Could you check a few things on this model? Use its own coordinates, in mm. A direction names the side the tool comes from. Coordinates: 2 decimals unless noted, no trailing zeros. Order: outer loops, then holes, each group sorted by start corner. A loop starts at its lowest first (then second) coordinate and runs counter-clockwise, first axis right, second up. Notation, with made-up numbers: (21, -33) -> (40, -33) arc R25 cw to (40, -21) -> close; hole circle Ø5 at (86.5, 51). An arc over 180 degrees is marked (long way). Put each result on its own line as item: value. Start each with the question number.
Q1. Please list where these lines run through material, in increasing order: line 1 along X through (y, z) = (-3, 7); line 2 along Z through (x, y) = (-6.5, -35.5); line 3 along X through (y, z) = (-43, 9).
Q2. For faces 4 (the face through (-23.2, 23.5, 10)), 5 (the face through (-40.1, 5, 2.7)), 6 (the face through (-46.6, 0.07, 9.14)), which set-ups out of +Z, -Z, +X, -X, +Y, -Y let a thin tool reach every point of the face, with its end or its side?
Q3. If we section it at B-B (x = 0): Please give me the cut outline in (y, z), and give its area (3 significant figures).
Q4. If we section it at D-D (x = 42): Please give me the cut outline in (y, z).
Q5. Will these pins go through, and if not, where does the flat tip stop? pin 1 (4 mm diameter, centred on x = -15, z = 8, fed in from +Y); pin 2 (8 mm diameter, centred on y = -42.33, z = 5, fed in from -X); pin 3 (8 mm diameter, centred on x = 21.5, z = 15, fed in from +Y); pin 4 (5.5 mm diameter, centred on x = 42.33, z = 5, fed in from -Y).
Q6. If we section it at A-A (z = 5): Count the separate pieces of the cut face and the enclosed holes in it, and give its area (3 significant figures).
Q7. We'd pull the mould along X, two halves only. Please class faces 1 (the face through (-0.07, 39.47, 5.9)), 2 (the face through (-25.14, -24.22, 12.07)), 3 (the face through (-20.98, -28.05, 13.45)): +X half, -X half, draft (parallel to the pull), parting line (faces both ways), or undercut.
from build123d import *
from build123d.topology import SkipClean

# Parameters (mm, degrees)
CROQUIS1_R                 = 32.5
SALIENTE_EXTRUIR1_DEPTH    = 10
CROQUIS2_R                 = 3
CORTAR_EXTRUIR1_DEPTH      = 72.50174823
MATRIZC1_COUNT             = 4
SALIENTE_EXTRUIR2_DEPTH    = 10
CORTAR_EXTRUIR2_DEPTH      = 71.089228844
CORTAR_EXTRUIR2_DEPTH_BACK = 71.089228844
CROQUIS4_R                 = 3
REDONDEO1_R                = 3
SIMETR_A3_START            = 32.113081288
SIMETR_A3_DEPTH            = 5.333547499
SIMETR_A3_START_2          = -5
SIMETR_A3_2_DEPTH          = 10
SIMETR_A3_3_DEPTH          = 10


# Read off the part's stored shape, not the designer's step: Simetría3
with BuildPart() as part:
    # Croquis1 → Saliente-Extruir1 (new body)
    with BuildSketch(Plane.XY):
        with BuildLine():
            Line((-5, 47.5), (5, 47.5))
            Line((5, 47.5), (5, 37.165171868))
            ThreePointArc((5, 37.165171868), (26.516504294, 26.516504294), (37.165171868, 5))
            Line((37.165171868, 5), (47.5, 5))
            Line((47.5, 5), (47.5, -5))
            Line((47.5, -5), (37.165171868, -5))
            ThreePointArc((37.165171868, -5), (26.516504294, -26.516504294), (5, -37.165171868))
            Line((5, -37.165171868), (5, -47.5))
            Line((5, -47.5), (-5, -47.5))
            Line((-5, -47.5), (-5, -37.165171868))
            ThreePointArc((-5, -37.165171868), (-26.516504294, -26.516504294), (-37.165171868, -5))
            Line((-37.165171868, -5), (-47.5, -5))
            Line((-47.5, -5), (-47.5, 5))
            Line((-47.5, 5), (-37.165171868, 5))
            ThreePointArc((-37.165171868, 5), (-26.516504294, 26.516504294), (-5, 37.165171868))
            Line((-5, 37.165171868), (-5, 47.5))
        make_face()
        Circle(CROQUIS1_R, mode=Mode.SUBTRACT)
    extrude(amount=SALIENTE_EXTRUIR1_DEPTH)

    # Croquis2 → Cortar-Extruir1 (cut, through all)
    with BuildSketch(Plane(origin=(5, 0, 0), x_dir=(0, 0, -1), z_dir=(1, 0, 0))):
        with Locations(Location((-5, -42.332585934, 0), (0, 0, 90))):
            Circle(CROQUIS2_R)
    cortar_extruir1 = extrude(amount=-CORTAR_EXTRUIR1_DEPTH, mode=Mode.SUBTRACT)

    # MatrizC1: Cortar-Extruir1 ×4 about axis
    matrizc1_axis = Axis((0, 0, 10), (0, 0, 1))
    for i in range(1, MATRIZC1_COUNT):
        add(cortar_extruir1.rotate(matrizc1_axis, i * 360 / MATRIZC1_COUNT), mode=Mode.SUBTRACT)

    # Croquis3 → Saliente-Extruir2 (add)
    with SkipClean():  # the faces are left unmerged after this step: merging them gives an invalid solid
        with BuildSketch(Plane.XY.offset(10)):
            with BuildLine():
                Line((19.17184375, 26.242911562), (22.744211146, 29.815278958))
                ThreePointArc((22.744211146, 29.815278958), (26.516504294, 26.516504294), (29.815278958, 22.744211146))
                Line((29.815278958, 22.744211146), (26.242911562, 19.17184375))
                ThreePointArc((26.242911562, 19.17184375), (22.980970389, 22.980970389), (19.17184375, 26.242911562))
            make_face()
            with BuildLine():
                Line((-26.242911562, -19.17184375), (-29.815278958, -22.744211146))
                ThreePointArc((-29.815278958, -22.744211146), (-26.516504294, -26.516504294), (-22.744211146, -29.815278958))
                Line((-22.744211146, -29.815278958), (-19.17184375, -26.242911562))
                ThreePointArc((-19.17184375, -26.242911562), (-22.980970389, -22.980970389), (-26.242911562, -19.17184375))
            make_face()
        extrude(amount=SALIENTE_EXTRUIR2_DEPTH)

    # Croquis4 → Cortar-Extruir2 (cut, two sides: drawn at the far end of the back side and taken through both)
    with SkipClean():  # the faces are left unmerged after this step: merging them gives an invalid solid
        with BuildSketch(Plane(origin=(0, 0, 0), x_dir=(-0.7071067811865476, 0.7071067811865475, 0), z_dir=(-0.7071067811865475, -0.7071067811865476, 0)).offset(-CORTAR_EXTRUIR2_DEPTH_BACK)):
            with Locations(Location((0, -15, 0), (0, 0, 180))):
                Circle(CROQUIS4_R)
        extrude(amount=CORTAR_EXTRUIR2_DEPTH + CORTAR_EXTRUIR2_DEPTH_BACK, mode=Mode.SUBTRACT)

    # Redondeo1
    redondeo1_edges = [part.edges().sort_by_distance(p)[0] for p in [
        (-47.5, 0, 10),
        (0, -47.5, 0),
        (-47.5, 0, 0),
        (0, -47.5, 10),
        (-28.02909526, -20.958027448, 20),
        (-20.958027448, -28.02909526, 20),
    ]]
    fillet(redondeo1_edges, radius=REDONDEO1_R)

    # Simetría3 outline → Simetría3 (cut)
    with SkipClean():  # the faces are left unmerged after this step: merging them gives an invalid solid
        with BuildSketch(Plane(origin=(0, 0, 0), x_dir=(0.707106781186546, -0.707106781186549, 0), z_dir=(0.707106781186549, 0.707106781186546, 0)).offset(SIMETR_A3_START)):
            with BuildLine():
                Line((-5, -20), (-2, -20))
                ThreePointArc((-2, -20), (-4.121320344, -19.121320344), (-5, -17))
                Line((-5, -17), (-5, -20))
            make_face()
            with BuildLine():
                ThreePointArc((5, -17), (4.121320344, -19.121320344), (2, -20))
                Line((2, -20), (5, -20))
                Line((5, -20), (5, -17))
            make_face()
        extrude(amount=SIMETR_A3_DEPTH, mode=Mode.SUBTRACT)

    # Simetr_a3 2 outline → Simetr_a3 2 (cut)
    with SkipClean():  # the faces are left unmerged after this step: merging them gives an invalid solid
        with BuildSketch(Plane.YZ.offset(SIMETR_A3_START_2)):
            with BuildLine():
                Line((47.5, 10), (44.5, 10))
                ThreePointArc((44.5, 10), (46.621320344, 9.121320344), (47.5, 7))
                Line((47.5, 7), (47.5, 10))
            make_face()
            with BuildLine():
                Line((47.5, 0), (47.5, 3))
                ThreePointArc((47.5, 3), (46.621320344, 0.878679656), (44.5, 0))
                Line((44.5, 0), (47.5, 0))
            make_face()
        extrude(amount=SIMETR_A3_2_DEPTH, mode=Mode.SUBTRACT)

    # Simetr_a3 3 outline → Simetr_a3 3 (cut)
    with SkipClean():  # the faces are left unmerged after this step: merging them gives an invalid solid
        with BuildSketch(Plane(origin=(0, 0, 0), x_dir=(1, 0, 0), z_dir=(0, 1, 0)).offset(SIMETR_A3_START_2)):
            with BuildLine():
                Line((47.5, 0), (44.5, 0))
                ThreePointArc((44.5, 0), (46.621320344, -0.878679656), (47.5, -3))
                Line((47.5, -3), (47.5, 0))
            make_face()
            with BuildLine():
                Line((47.5, -10), (47.5, -7))
                ThreePointArc((47.5, -7), (46.621320344, -9.121320344), (44.5, -10))
                Line((44.5, -10), (47.5, -10))
            make_face()
        extrude(amount=SIMETR_A3_3_DEPTH, mode=Mode.SUBTRACT)


solid = part.part
The answers:
1. line 1: -47.5 to -44.57, -40.1 to -32.36, 32.36 to 40.1, 44.57 to 47.5
1. line 2: 0 to 10
1. line 3: -5 to 5
2. face 4: +Z, -X, +Y
2. face 5: +Z, -Z, -X, +Y
2. face 6: +Z, -X, +Y, -Y
3. outline: (-47.5, 3) arc R3 ccw to (-44.5, 0) -> (-32.5, 0) -> (-32.5, 10) -> (-44.5, 10) arc R3 ccw to (-47.5, 7) -> close; (32.5, 0) -> (44.5, 0) arc R3 ccw to (47.5, 3) -> (47.5, 7) arc R3 ccw to (44.5, 10) -> (32.5, 10) -> close; hole circle Ø6 at (-42.33, 5); hole circle Ø6 at (42.33, 5)
3. area: 236 mm^2
4. outline: (-5, 0) -> (5, 0) -> (5, 2.02) -> (-5, 2.02) -> close; (-5, 7.98) -> (5, 7.98) -> (5, 10) -> (-5, 10) -> close
5. pin 1: y = 35.17
5. pin 2: x = -5
5. pin 3: y = 29.82
5. pin 4: through
6. separate pieces: 5
6. enclosed holes: 1
6. area: 1,260 mm^2
7. face 1: draft
7. face 2: undercut
7. face 3: +X half
